Autodesk Inventor part; units mm, degrees
ref_plane "YZ Plane" through (0, 0, 0) normal (1, 0, 0) x (0, 1, 0)
ref_plane "XZ Plane" through (0, 0, 0) normal (0, 1, 0) x (-1, 0, 0)
ref_plane "XY Plane" through (0, 0, 0) normal (0, 0, 1) x (1, 0, 0)
sketch "Sketch_1" plane through (0, 0, 0) normal (0, 0, 1) x (1, 0, 0)
  line L0 (130, 0) -> (0, 0)
  line L1 (0, 0) -> (0, 3.5)
  line L2 (0, 3.5) -> (0.5, 4)
  line L3 (0.5, 4) -> (129.5, 4)
  line L4 (129.5, 4) -> (130, 3.5)
  line L5 (130, 3.5) -> (130, 0)
  line L6 (130, 0) -> (0, 0)
revolve "Revolution1" add sketch "Sketch_1" angle 360 about axis through (130, 0, 0) along (1, 0, 0)
sketch "Sketch2" plane through (0, 0, 0) normal (-1, 0, 0) x (0, 0, 1)
  point P0 (0, 0)
hole "Hole1" at (0, 0, 0) direction (1, 0, 0) diameter 2.459 depth 8.2901 tip angle 120 countersink diameter 3 countersink angle 90
sketch "Sketch3" plane through (130, 0, 0) normal (1, 0, 0) x (0, 0, -1)
  point P0 (0, 0)
hole "Hole2" at (130, 0, 0) direction (-1, 0, 0) diameter 2.459 depth 8.2901 tip angle 120 countersink diameter 3 countersink angle 90
properties part number "AETTF8-130-M3-N3"
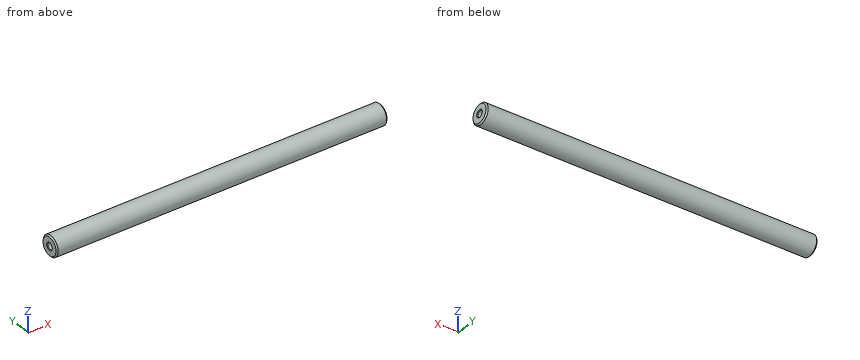
Here's how the part is built. I have some questions about the finished solid (model axes, mm). Coordinates: 2 decimals unless noted, no trailing zeros. Order: outer loops, then holes, each group sorted by start corner. A loop starts at its lowest first (then second) coordinate and runs counter-clockwise, first axis right, second up. Notation, with made-up numbers: (27, 85) - (86, 85) arc R5 cw to (86, 94) - close; hole circle Ø6 at (-8.75, 7). An arc over 180 degrees is marked (long way). One line per question, with ' | ' between items. Start each with the question number.
1. I'm going to push flat-ended pins straight in: pin 1 Ø3 at (x, y) = (90, -2.5) entering from -Z; pin 2 Ø2 at (x, y) = (113, -2) entering from +Z; pin 3 Ø3 at (x, z) = (75.5, 3) entering from +Y. Where does each tip first touch, or does it pass through?
2. Please list where these lines run through material, in increasing order: line 1 along Z through (x, y) = (125, 0); line 2 along Z through (x, y) = (105, -0.25); line 3 along Y through (x, z) = (81, 3.25). Write a range as [from, to].
3. If we section it at A-A (x = 48): Write out the boundary of the cut face in (y, z).
Model answer:
1) pin 1: stops at z = -3.87 | pin 2: stops at z = 3.87 | pin 3: stops at y = 3.71
2) line 1: z = [-4, -1.23], [1.23, 4] | line 2: z = [-3.99, 3.99] | line 3: y = [-2.33, 2.33]
3) outline: circle Ø8 at (0, 0)
